Work out the finished part from the listing and answer in its coordinate system (mm). A direction names the side the tool comes from. Round coordinates to 2 decimals unless told otherwise and drop trailing zeros. Order: outer loops, then holes, each group sorted by start corner. A loop starts at its lowest first (then second) coordinate and runs counter-clockwise, first axis right, second up. Notation, with made-up numbers: (42, 0) - (97, 0) arc R7 cw to (97, 10) - close; hole circle Ø3 at (55.25, 78.25). An arc over 180 degrees is marked (long way). Answer in a Markdown table with one row per item.
from build123d import *

# Parameters (mm, degrees)
SKETCH1_R           = 35
BOSS_EXTRUDE1_DEPTH = 30
SKETCH2_R           = 10
CUT_EXTRUDE1_DEPTH  = 30


with BuildPart() as part:
    # Sketch1 → Boss-Extrude1 (new body)
    with BuildSketch(Plane(origin=(0, 0, 0), x_dir=(0, 0, -1), z_dir=(1, 0, 0))):
        with BuildLine():
            Line((0, -45), (80, -45))
            Line((80, -45), (80, -35))
            Line((80, -35), (28.284271247, -35))
            ThreePointArc((28.284271247, -35), (0, 45), (-28.284271247, -35))
            Line((-28.284271247, -35), (-80, -35))
            Line((-80, -35), (-80, -45))
            Line((-80, -45), (0, -45))
        make_face()
        Circle(SKETCH1_R, mode=Mode.SUBTRACT)
    extrude(amount=BOSS_EXTRUDE1_DEPTH)

    # Sketch2 → Cut-Extrude1 (cut)
    with BuildSketch(Plane(origin=(0, -35, 0), x_dir=(1, 0, 0), z_dir=(0, 1, 0))):
        with Locations(Location((15, 62.399384691, 0), (0, 0, 270))):
            Circle(SKETCH2_R)
        with Locations(Location((15, -62.600615309, 0), (0, 0, 270))):
            Circle(SKETCH2_R)
    extrude(amount=-CUT_EXTRUDE1_DEPTH, mode=Mode.SUBTRACT)


solid = part.part
1) Which of the six approach directions +Z, -Z, +X, -X, +Y, -Y give full straight-line access (tool end or side, diameter ignored) to faces 4 (the face through (18, -39.93, -52.86)), 5 (the face through (15, -35, 48)), 6 (the face through (15, -35, -49))?
Filled in:
| item | result |
|---|---|
| face 4 | +Y, -Y |
| face 5 | +Z, +X, -X |
| face 6 | -Z, +X, -X |
2) Find section A-A, the plane x = 15. Give the vertices of the cut face in (y, z), then the cut area to 3 significant figures.
Filled in:
| item | result |
|---|---|
| outline | (-45, -80) - (-35, -80) - (-35, -72.4) - (-45, -72.4) - close; (-45, -52.4) - (-35, -52.4) - (-35, -28.28) arc R45 ccw (long way) to (-35, 28.28) - (-35, 52.6) - (-45, 52.6) - close; (-45, 72.6) - (-35, 72.6) - (-35, 80) - (-45, 80) - close; hole circle Ø70 at (0, 0) |
| area | 3,330 mm^2 |
3) Each of these flat-tipped pins is pushed along its axis until it touches: pin 1 (15 mm diameter, centred on x = 9, z = -66.5, fed in from +Y); pin 2 (8 mm diameter, centred on x = 22.5, y = 35.5, fed in from -Z); pin 3 (3 mm diameter, centred on x = 13.5, z = -26.5, fed in from +Y). Where does it stop, or does it pass through?
Filled in:
| item | result |
|---|---|
| pin 1 | stops at y = -35 |
| pin 2 | stops at z = -32.14 |
| pin 3 | stops at y = 37.42 |
4) The mould has two halves that part along Y. Classify faces 1 (the face through (15, -40, -80)), 2 (the face through (15, -45, 1)), 3 (the face through (14.79, 44.973, -1.551)): released by +Y, released by -Y, zero draft, split by the parting line, or undercut.
Filled in:
| item | result |
|---|---|
| face 1 | zero draft |
| face 2 | released by -Y |
| face 3 | undercut |
5) Find the intervals of material crossed by probe 1 along Y at (x, z) = (4.5, -1); probe 2 along Z at (x, y) = (18.5, 32.5); probe 3 along Z at (x, y) = (28, 32), in increasing order. Write a range as from..to.
Filled in:
| item | result |
|---|---|
| probe 1 | y = -45..-34.99, 34.99..44.99 |
| probe 2 | z = -31.12..-12.99, 12.99..31.12 |
| probe 3 | z = -31.64..-14.18, 14.18..31.64 |
6) Find section B-B, the plane z = 0. Give the vertices of the cut face in (x, y), then the cut area to 3 significant figures.
Filled in:
| item | result |
|---|---|
| outline | (0, -45) - (30, -45) - (30, -35) - (0, -35) - close; (0, 35) - (30, 35) - (30, 45) - (0, 45) - close |
| area | 600 mm^2 |
7) Find section C-C, the plane y = -15. Give the vertices of the cut face in (x, z).
Filled in:
| item | result |
|---|---|
| outline | (0, -42.43) - (30, -42.43) - (30, -31.62) - (0, -31.62) - close; (0, 31.62) - (30, 31.62) - (30, 42.43) - (0, 42.43) - close |
8) Find section D-D, the plane x = 6.5. Give the vertices of the cut face in (y, z).
Filled in:
| item | result |
|---|---|
| outline | (-45, -80) - (-35, -80) - (-35, -67.67) - (-45, -67.67) - close; (-45, -57.13) - (-35, -57.13) - (-35, -28.28) arc R45 ccw (long way) to (-35, 28.28) - (-35, 57.33) - (-45, 57.33) - close; (-45, 67.87) - (-35, 67.87) - (-35, 80) - (-45, 80) - close; hole circle Ø70 at (0, 0) |
